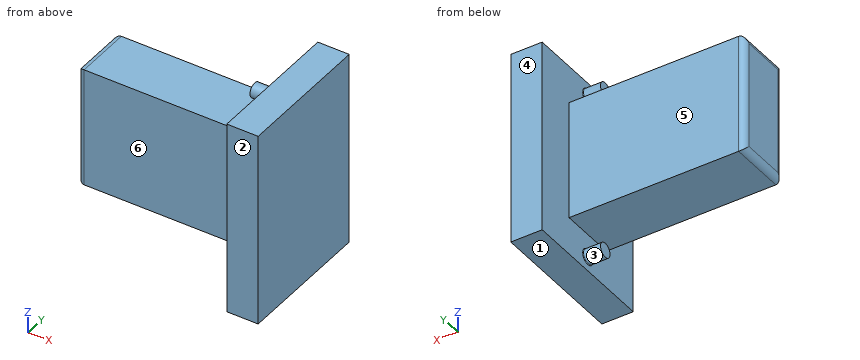
from build123d import *

# Parameters (mm, degrees)
SKETCH1_W           = 31
SKETCH1_H           = 22
BOSS_EXTRUDE1_DEPTH = 5
SKETCH2_W           = 19
SKETCH2_H           = 9
BOSS_EXTRUDE2_DEPTH = 28
FILLET1_R           = 1
SKETCH3_R           = 1.15
BOSS_EXTRUDE3_DEPTH = 2.8
FILLET2_R           = 0.1
SKETCH4_R           = 1.15
BOSS_EXTRUDE4_DEPTH = 2.8
FILLET3_R           = 0.1


with BuildPart() as part:
    # Sketch1 → Boss-Extrude1 (new body)
    with BuildSketch(Plane(origin=(0, 0, 0), x_dir=(0, 0, -1), z_dir=(1, 0, 0))):
        with Locations((15.5, 11)):
            Rectangle(SKETCH1_W, SKETCH1_H)
    extrude(amount=BOSS_EXTRUDE1_DEPTH)

    # Sketch2 → Boss-Extrude2 (add)
    with BuildSketch(Plane.ZY):
        with Locations((-15.5, 11)):
            Rectangle(SKETCH2_W, SKETCH2_H)
    extrude(amount=BOSS_EXTRUDE2_DEPTH)

    # Fillet1
    fillet1_edges = [part.edges().sort_by_distance(p)[0] for p in [
        (-28, 11, -25),
        (-28, 6.5, -15.5),
        (-28, 11, -6),
        (-28, 15.5, -15.5),
    ]]
    fillet(fillet1_edges, radius=FILLET1_R)

    # Sketch3 → Boss-Extrude3 (add)
    with BuildSketch(Plane.ZY):
        with Locations((-2.25, 11)):
            Circle(SKETCH3_R)
    extrude(amount=BOSS_EXTRUDE3_DEPTH)

    # Fillet2
    fillet2_edges = [part.edges().sort_by_distance(p)[0] for p in [
        (0, 11, -3.4),
    ]]
    fillet(fillet2_edges, radius=FILLET2_R)

    # Sketch4 → Boss-Extrude4 (add)
    with BuildSketch(Plane.ZY):
        with Locations((-28.75, 11)):
            Circle(SKETCH4_R)
    extrude(amount=BOSS_EXTRUDE4_DEPTH)

    # Fillet3
    fillet3_edges = [part.edges().sort_by_distance(p)[0] for p in [
        (0, 11, -29.9),
    ]]
    fillet(fillet3_edges, radius=FILLET3_R)


solid = part.part
Input: part model. Units: mm. Frame: model coordinates. Face numbers are marked on the shaded views. A direction names the side the tool comes from. Give positions to 0.01 mm unless a question says otherwise; leave off trailing zeros. Order: outer loops, then holes, each group sorted by start corner. A loop starts at its lowest first (then second) coordinate and runs counter-clockwise, first axis right, second up. Notation, with made-up numbers: (43.5, 88.25) - (65.5, 88.25) arc R18 cw to (65.5, 95.25) - close; hole circle Ø4 at (-3.75, 36.5). An arc over 180 degrees is marked (long way). Answer as a JSON object with one key per item and string values. Group by question number.
Q1. Cut plane D-D, the plane z = -19.5. Output: boundary loops of the cut face in (x, y).
Q2. Cut plane A-A, the plane z = -2.25. Output: boundary loops of the cut face in (x, y).
Q3. Mould query, pull axis Z, two halves, no side actions, for the marked faces 1, 2 and 3. Classes: pulls with the +Z half, pulls with the -Z half, needs draft (parallel to the pull), parting line crosses it, or undercut.
Q4. Line query: probe 1 along X at (y, z) = (3.75, -14); probe 2 along Y at (x, z) = (-25.5, -7); probe 3 along Z at (x, y) = (-9, 9.5). Output: solid intervals per line, ascending.
Q5. Set-up query: the marked faces 4, 5 and 6. Return all of +Z, -Z, +X, -X, +Y, -Y with unobstructed straight access to the full face (end or side cutting, diameter ignored); none if empty.
Q6. First-contact query: pin 1 Ø5 at (x, y) = (-16.5, 5) entering from -Z; pin 2 Ø9.5 at (x, z) = (-15.5, -17) entering from -Y; pin 3 Ø1.5 at (x, y) = (-7, 11.5) entering from +Z. Flat tips, straight axial feed; report the tip coordinate or a pass-through.
Q7. Cut plane B-B, the plane y = 11. Output: boundary loops of the cut face in (x, z).
Q8. Cut plane C-C, the plane x = -7. Output: boundary loops of the cut face in (y, z), then the cut area to 3 significant figures.
Results:
{
 "1": {"outline": "(-28, 7.5) arc R1 ccw to (-27, 6.5) - (0, 6.5) - (0, 0) - (5, 0) - (5, 22) - (0, 22) - (0, 15.5) - (-27, 15.5) arc R1 ccw to (-28, 14.5) - close"},
 "2": {"outline": "(-2.8, 9.85) - (-0.1, 9.85) arc R0.1 cw to (0, 9.75) - (0, 0) - (5, 0) - (5, 22) - (0, 22) - (0, 12.25) arc R0.1 cw to (-0.1, 12.15) - (-2.8, 12.15) - close"},
 "3": {"face 1": "pulls with the -Z half", "face 2": "needs draft", "face 3": "undercut"},
 "4": {"probe 1": "0 to 5", "probe 2": "6.5 to 15.5", "probe 3": "-25 to -6"},
 "5": {"face 4": "+Z, -Z, +X, -X, +Y", "face 5": "+Z, -Z, -X, +Y", "face 6": "+Z, -Z, -X, -Y"},
 "6": {"pin 1": "z = -25", "pin 2": "y = 6.5", "pin 3": "z = -6"},
 "7": {"outline": "(-28, -24) arc R1 ccw to (-27, -25) - (0, -25) - (0, -27.5) arc R0.1 cw to (-0.1, -27.6) - (-2.8, -27.6) - (-2.8, -29.9) - (-0.1, -29.9) arc R0.1 cw to (0, -30) - (0, -31) - (5, -31) - (5, 0) - (0, 0) - (0, -1) arc R0.1 cw to (-0.1, -1.1) - (-2.8, -1.1) - (-2.8, -3.4) - (-0.1, -3.4) arc R0.1 cw to (0, -3.5) - (0, -6) - (-27, -6) arc R1 ccw to (-28, -7) - close"},
 "8": {"outline": "(6.5, -25) - (15.5, -25) - (15.5, -6) - (6.5, -6) - close", "area": "171 mm^2"}
}
